from build123d import *

# Parameters (mm, degrees)
F1_W     = 14.673665
F1_H     = 14.677159
F2_DEPTH = 11.43
F3_R     = 2.823757
F3_R_2   = 2.731621
F3_R_3   = 3.000674
F5_DEPTH = 3.556


with BuildPart() as f2:
    # F1 (on face) → F2 (new body)
    with BuildSketch(Plane.XY):
        with Locations((-181.473411, -79.122174)):
            Rectangle(F1_W, F1_H)
    extrude(amount=F2_DEPTH)

    # F3 (on face) → F5 (join)
    with BuildSketch(Plane.XY.offset(11.43)):
        with BuildLine():
            ThreePointArc((-178.254932, -71.783595), (-180.231409, -76.555231), (-175.459772, -74.578755))
            ThreePointArc((-175.459772, -74.578755), (-176.278456, -72.602278), (-178.254932, -71.783595))
        make_face()
        with Locations((-178.254932, -82.677774)):
            Circle(F3_R)
        with Locations((-184.495822, -74.578755)):
            Circle(F3_R_2)
        with Locations((-184.46213, -82.193248)):
            Circle(F3_R_3)
    extrude(amount=F5_DEPTH)


solid = f2.part
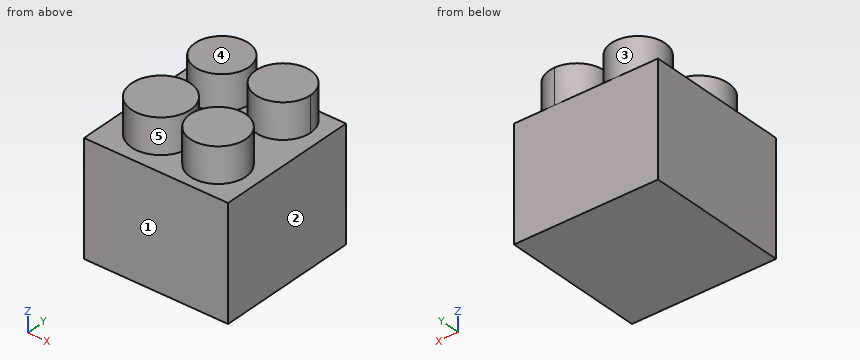
Design review of the part built by this model. Coordinates are the model's own, in mm. Face numbers are marked on the shaded views. A direction names the side the tool comes from. Round coordinates to 2 decimals unless told otherwise and drop trailing zeros. Write each loop counter-clockwise with the first axis right and the second up, starting at its lowest first coordinate (ties: lowest second). Pieces come first, ordered by that corner, then holes.
Item 1: Draft analysis for pull direction Y (two halves, no side actions). For the marked faces 1, 2 and 3, state which applies: released by +Y, released by -Y, zero draft, split by the parting line, or undercut.
Item 2: Consider section D-D on y = -78.75. Give the boundary of the cut face in (x, z).
Item 3: Wall thickness on L1, parallel to Z at x = -183, y = -77.75; L2, parallel to X at y = -73.5, z = 12; L3, parallel to Y at x = -186, z = 13.75: over which ranges is each line inside the solid? List them lowest first.
Item 4: Consider section C-C on x = -174.75. Give the boundary of the cut face in (y, z).
Item 5: For the marked faces 4 and 5, list the 3-axis set-ups (+Z, -Z, +X, -X, +Y, -Y) from which the entire face can be reached by the end or side of a thin tool; tool diameter is ignored.
Item 6: Consider section A-A on y = -73.5. Give the boundary of the cut face in (x, z).
Check values:
1. face 1: released by -Y
1. face 2: zero draft
1. face 3: undercut
2. outline: (-188.81, 0) - (-174.14, 0) - (-174.14, 11.43) - (-188.81, 11.43) - close
3. L1: z = 0 to 11.43
3. L2: x = -187.01 to -181.99, -180.83 to -175.68
3. L3: y = -84.77 to -79.62, -76.86 to -72.3
4. outline: (-86.46, 0) - (-71.78, 0) - (-71.78, 11.43) - (-86.46, 11.43) - close
5. face 4: +Z, +X, -X, +Y, -Y
5. face 5: +Z
6. outline: (-188.81, 0) - (-174.14, 0) - (-174.14, 11.43) - (-175.68, 11.43) - (-175.68, 14.99) - (-180.83, 14.99) - (-180.83, 11.43) - (-181.99, 11.43) - (-181.99, 14.99) - (-187.01, 14.99) - (-187.01, 11.43) - (-188.81, 11.43) - close
